from build123d import *

# Parameters (mm, degrees)
F1_DEPTH = 3


with BuildPart() as f1:
    # F0 (on Top) → F1 (new body)
    with BuildSketch(Plane.XY):
        with BuildLine():
            ThreePointArc((15.716234, 0), (13.804101, 0.688345), (12.76944, 2.4375))
            ThreePointArc((12.76944, 2.4375), (-1.22419, 12.942232), (-13, 0))
            ThreePointArc((-13, 0), (-1.125, -11.875), (10.75, 0))
            ThreePointArc((10.75, 0), (0, 10.75), (-10.75, 0))
            ThreePointArc((-10.75, 0), (-2.707419, -9.599334), (8.151994, -3.362069))
            ThreePointArc((8.151994, -3.362069), (7.85535, -1.069121), (5.805329, 0))
            Line((5.805329, 0), (2.75, 0))
            Line((2.75, 0), (2.75, -1.2))
            Line((2.75, -1.2), (5.876591, -1.2))
            ThreePointArc((5.876591, -1.2), (6.898085, -1.729549), (7.054089, -2.869521))
            ThreePointArc((7.054089, -2.869521), (-2.456028, -8.42511), (-9.55, 0))
            ThreePointArc((-9.55, 0), (0, 9.55), (9.55, 0))
            ThreePointArc((9.55, 0), (-1.125, -10.675), (-11.8, 0))
            ThreePointArc((-11.8, 0), (-1.111188, 11.747564), (11.590722, 2.2125))
            ThreePointArc((11.590722, 2.2125), (13.039248, -0.236317), (15.716234, -1.2))
            Line((15.716234, -1.2), (18, -1.2))
            Line((18, -1.2), (18, 0))
            Line((18, 0), (15.716234, 0))
        make_face()
    extrude(amount=F1_DEPTH)


solid = f1.part
Build history of the part. All positions in model axes, mm. A direction names the side the tool comes from. Round coordinates to 2 decimals unless told otherwise and drop trailing zeros. Loops run counter-clockwise (first coordinate to the right, second up) from the corner with the lowest first, then second, coordinate; pieces in that order, holes last. Notation, with made-up numbers: (88.25, 24.5) -> (145.25, 24.5) arc R11 cw to (145.25, 30.5) -> close; hole circle Ø11 at (53, 2.5). An arc over 180 degrees is marked (long way). Use CSV: the item, a comma, the result in double quotes. Start each with the question number.
Q1. Which spindle directions (+Z, -Z, +X, -X, +Y, -Y) get a long thin tool onto all of the face, cutting with end or side? Do faces 4 (the face through (17, 0, 1)), 5 (the face through (13.01, -0.21, 1.48)), 6 (the face through (-1.354, 11.722, 1.479)). Say none if no direction does.
Q2. Flat gauge pins, fed straight in: pin 1 Ø10 at (x, y) = (3, -5.5) entering from -Z; pin 2 Ø0.9 at (x, z) = (5, 1.5) entering from -Y. Where does each tip first touch, or does it go through?
Q3. Saw through at A-A on x = -7. Give the cut face in (y, z), and give its area (3 significant figures).
Q4. Saw through at B-B on y = 8.5. Give the cut face in (x, z), and give its area (3 significant figures).
Q5. Drill centre lines: L1, parallel to Y at x = -4, z = 2.1; L2, parallel to Y at x = -2.5, z = 1.6; L3, parallel to X at y = -4.5, z = 0.6. Where is each one in solid material? Low to high.
Q6. Mould opens along Y. For faces 1 (the face through (18, -1, 1)), 2 (the face through (13.827, 0.67, 1.479)), 3 (the face through (0.236, 10.747, 1.479)) say: +Y half, -Y half, draft (parallel to the pull), parting line (faces both ways), or undercut.
Solutions:
1,face 4,"+Z, -Z, +X, +Y"
1,face 5,"+Z, -Z, -Y"
1,face 6,"+Z, -Z"
2,pin 1,"stops at z = 0"
2,pin 2,"stops at y = -10.43"
3,outline,"(-10.32, 0) -> (-8.91, 0) -> (-8.91, 3) -> (-10.32, 3) -> close; (-7.69, 0) -> (-6.09, 0) -> (-6.09, 3) -> (-7.69, 3) -> close; (6.5, 0) -> (8.16, 0) -> (8.16, 3) -> (6.5, 3) -> close; (9.5, 0) -> (10.95, 0) -> (10.95, 3) -> (9.5, 3) -> close"
3,area,"18.4 mm^2"
4,outline,"(-9.84, 0) -> (-8.18, 0) -> (-8.18, 3) -> (-9.84, 3) -> close; (-6.58, 0) -> (-4.35, 0) -> (-4.35, 3) -> (-6.58, 3) -> close; (4.35, 0) -> (6.58, 0) -> (6.58, 3) -> (4.35, 3) -> close; (8.18, 0) -> (9.84, 0) -> (9.84, 3) -> (8.18, 3) -> close"
4,area,"23.3 mm^2"
5,L1,"y = -11.52 to -10.28, -9.28 to -8.01, 8.67 to 9.98, 11.1 to 12.37"
5,L2,"y = -11.8 to -10.59, -9.63 to -8.42, 9.22 to 10.46, 11.53 to 12.76"
5,L3,"x = -12.11 to -10.81, -9.65 to -8.27, 6.27 to 7.65, 8.56 to 9.86"
6,face 1,"draft"
6,face 2,"+Y half"
6,face 3,"undercut"
